Geometry check sheet. Reference: the model listing, model coordinates, mm. A direction names the side the tool comes from. Give positions to 0.01 mm unless a question says otherwise; leave off trailing zeros. Write each loop counter-clockwise with the first axis right and the second up, starting at its lowest first coordinate (ties: lowest second). Pieces come first, ordered by that corner, then holes. Notation, with made-up numbers: (-36, 46) - (-21, 46) arc R8 ccw to (-21, 57) - close; hole circle Ø3 at (72, 27.25). An arc over 180 degrees is marked (long way). Use a Markdown table: item, result.
Autodesk Inventor part; units mm, degrees
ref_plane "YZ Plane" through (0, 0, 0) normal (1, 0, 0) x (0, 1, 0)
ref_plane "XZ Plane" through (0, 0, 0) normal (0, 1, 0) x (-1, 0, 0)
ref_plane "XY Plane" through (0, 0, 0) normal (0, 0, 1) x (1, 0, 0)
sketch "Sketch1" plane through (0, 0, 0) normal (1, 0, 0) x (0, 1, 0)
  line L0 (-12.7, 12.7) -> (0, 12.7)
  line L1 (12.7, 0) -> (12.7, -12.7)
  line L2 (12.7, -12.7) -> (-12.7, -12.7)
  line L3 (-12.7, -12.7) -> (-12.7, 12.7)
  line L4 (-12.7, 12.7) -> (12.7, -12.7) construction
  line L5 (0, 0) -> (-12.7, -12.7) construction
  line L6 (0, 0) -> (12.7, 0)
  line L7 (0, 12.7) -> (0, 0)
  line L8 (12.7, 0) -> (0, 0)
  dimension "d0" = 25.4
extrude "Extrusion1" add sketch "Sketch1" along normal mid plane 19.05
ref_plane "Work Plane2" through (29.3294, 29.3294, 29.3294) normal (0.5774, 0.5774, 0.5774) x (0.7071, 0, -0.7071)
ref_plane "Work Plane1" through (0, 0, 0) normal (0.5774, 0.5774, 0.5774) x (0.7071, 0, -0.7071)
sketch "Sketch2" plane through (29.3294, 29.3294, 29.3294) normal (0.5774, 0.5774, 0.5774) x (0.7071, 0, -0.7071)
  line L0 (-6.7352, 14.2581) -> (6.7352, 6.4809) construction
  line L1 (15.7154, 11.6657) -> (6.7352, 6.4809) construction
  line L2 (2.2451, 19.4428) -> (15.7154, 11.6657) construction
  line L3 (-6.7352, 14.2581) -> (2.2451, 19.4428) construction
  line L4 (-6.7352, 3.8886) -> (6.7352, -3.8886) construction
  line L5 (6.7352, 6.4809) -> (6.7352, -3.8886) construction
  line L6 (-6.7352, 14.2581) -> (6.7352, 6.4809) construction
  line L7 (-6.7352, 3.8886) -> (-6.7352, 14.2581) construction
  line L8 (-2.2451, -9.0733) -> (-15.7154, -1.2962) construction
  line L9 (6.7352, -3.8886) -> (-2.2451, -9.0733) construction
  line L10 (-6.7352, 3.8886) -> (6.7352, -3.8886) construction
  line L11 (-15.7154, -1.2962) -> (-6.7352, 3.8886) construction
  line L12 (-15.7154, -11.6657) -> (-2.2451, -19.4428) construction
  line L13 (-2.2451, -9.0733) -> (-2.2451, -19.4428) construction
  line L14 (-2.2451, -9.0733) -> (-15.7154, -1.2962) construction
  line L15 (-15.7154, -11.6657) -> (-15.7154, -1.2962) construction
  line L16 (-2.2451, -9.0733) -> (-2.2451, -19.4428) construction
  line L17 (-2.2451, -19.4428) -> (15.7154, -9.0733) construction
  line L18 (15.7154, -9.0733) -> (15.7154, 11.6657) construction
  line L19 (15.7154, 11.6657) -> (6.7352, 6.4809) construction
  line L20 (6.7352, 6.4809) -> (6.7352, -3.8886) construction
  line L21 (6.7352, -3.8886) -> (-2.2451, -9.0733) construction
  line L22 (6.7352, 6.7742) -> (-6.2272, 14.2581)
  line L23 (-6.2272, 14.2581) -> (2.2451, 19.1495)
  line L24 (2.2451, 19.1495) -> (15.2074, 11.6657)
  line L25 (15.2074, 11.6657) -> (6.7352, 6.7742)
  line L26 (-6.4812, 13.8181) -> (6.4812, 6.3343)
  line L27 (6.4812, 6.3343) -> (6.4812, -3.4486)
  line L28 (6.4812, -3.4486) -> (-6.4812, 4.0352)
  line L29 (-6.4812, 4.0352) -> (-6.4812, 13.8181)
  line L30 (-6.7352, 3.5953) -> (6.2272, -3.8886)
  line L31 (6.2272, -3.8886) -> (-2.2451, -8.78)
  line L32 (-2.2451, -8.78) -> (-15.2074, -1.2962)
  line L33 (-15.2074, -1.2962) -> (-6.7352, 3.5953)
  line L34 (-15.4614, -1.7361) -> (-2.4991, -9.22)
  line L35 (-2.4991, -9.22) -> (-2.4991, -19.0029)
  line L36 (-2.4991, -19.0029) -> (-15.4614, -11.519)
  line L37 (-15.4614, -11.519) -> (-15.4614, -1.7361)
  line L38 (15.4614, 11.2258) -> (15.4614, -8.9267)
  line L39 (15.4614, -8.9267) -> (-1.9911, -19.0029)
  line L40 (-1.9911, -19.0029) -> (-1.9911, -9.22)
  line L41 (-1.9911, -9.22) -> (6.9892, -4.0352)
  line L42 (6.9892, -4.0352) -> (6.9892, 6.3343)
  line L43 (6.9892, 6.3343) -> (15.4614, 11.2258)
  point P0 (0, 0)
  dimension "d5" = 0.254
  dimension "d6" = 0.254
  dimension "d7" = 0.254
  dimension "d8" = 0.254
  dimension "d9" = 0.254
equation "\"d5\" = 0.5 * spacing"
equation "\"d6\" = 0.5 * spacing"
equation "\"d7\" = 0.5 * spacing"
equation "\"d8\" = 0.5 * spacing"
equation "\"d9\" = 0.5 * spacing"
equation "\"spacing\" = 0.508"
properties part number "iso"
1) Section check B-B on y = 7. Record the boundary of the cut face in (x, z) (3 decimals), then the cut area to 3 significant figures.
Working result:
| item | result |
|---|---|
| outline | (-9.525, -12.7) - (9.525, -12.7) - (9.525, 0) - (-9.525, 0) - close |
| area | 242 mm² |
2) Material ranges on L1, parallel to Z at x = 1.75, y = 9.5, recorded low to high. Write a range as from..to.
Working result:
| item | result |
|---|---|
| L1 | z = -12.7..0 |
3) Set-up check for faces 1 (the flat face through (0, 0, 6)), 2 (the flat face through (-9.525, -3, -3)): record each of +Z, -Z, +X, -X, +Y, -Y from which the full face is reachable in a straight line by a thin tool's end or side.
Working result:
| item | result |
|---|---|
| face 1 | +Z, +X, -X, +Y |
| face 2 | +Z, -Z, -X, +Y, -Y |
4) Depth check by flat-ended pin: P1, Ø10, axis at x = 4, y = 8, coming from the +Z side; P2, Ø6, axis at x = -1.5, z = 0.5, coming from the +Y side; P3, Ø4, axis at x = -1, z = 7.5, coming from the +Y side. Enter the tip coordinate at first touch or a pass-through.
Working result:
| item | result |
|---|---|
| P1 | stops at z = 0 |
| P2 | stops at y = 12.7 |
| P3 | stops at y = 0 |
5) Section check A-A on x = -5. Record the boundary of the cut face in (y, z), then the cut area to 3 significant figures.
Working result:
| item | result |
|---|---|
| outline | (-12.7, -12.7) - (12.7, -12.7) - (12.7, 0) - (0, 0) - (0, 12.7) - (-12.7, 12.7) - close |
| area | 484 mm² |
